CAD build for the part. Positions are in the model's coordinates, mm. Face numbers are marked on the shaded views. A direction names the side the tool comes from. Coordinates: 2 decimals unless noted, no trailing zeros. Loops run counter-clockwise (first coordinate to the right, second up) from the corner with the lowest first, then second, coordinate; pieces in that order, holes last. Notation, with made-up numbers: (-19, 74.25) -> (38, 74.25) arc R23 ccw to (38, 82.25) -> close; hole circle Ø7 at (8, -12). An arc over 180 degrees is marked (long way). Return JSON: item names as keys, results as strings. Group by question number.
(1) Probe L1, parallel to Z at x = 0, y = -0.7; L2, parallel to Z at x = 0, y = 0.6; L3, parallel to Y at x = -5, z = 0.75. List the from-to ranges inside material, lowest first.
(2) Tool access for the marked faces 4 and 5: list every direction of +Z, -Z, +X, -X, +Y, -Y with a clear straight run to the whole face (end or side of a thin tool).
(3) Mould opens along X. For the marked faces 1, 2 and 3 say: pulls with the +X half, pulls with the -X half, needs draft (parallel to the pull), parting line crosses it, or undercut.
(4) Saw through at C-C on y = 0.55. Write the cut outline in (x, z).
(5) Saw through at A-A on z = 0. Write the cut outline in (x, y).
(6) Flat gauge pins, fed straight in: pin 1 Ø1.5 at (x, y) = (-0.5, 0) entering from -Z; pin 2 Ø2 at (x, z) = (0, 0) entering from -Y. Where does each tip first touch, or does it go through?
(7) Saw through at B-B on x = 0. Write the cut outline in (y, z), then the cut area to 3 significant figures.
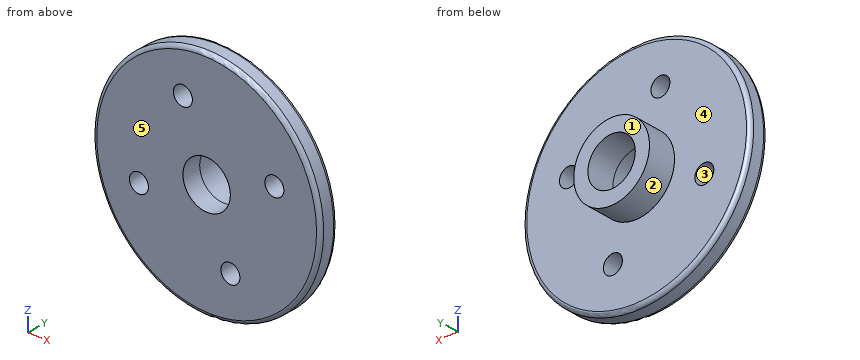
```python
from build123d import *

# Parameters (mm, degrees)
F0_R     = 6
F0_R_2   = 0.5
F0_R_3   = 1.25
F1_DEPTH = 1
F2_R     = 0.2
F3_R     = 2
F3_R_2   = 1.25
F4_DEPTH = 1.5


with BuildPart() as f1:
    # F0 (on Front) → F1 (new body)
    with BuildSketch(Plane.XZ):
        Circle(F0_R)
        with Locations((-3.573598, -1.254015)):
            Circle(F0_R_2, mode=Mode.SUBTRACT)
        with Locations((1.254015, -3.573598)):
            Circle(F0_R_2, mode=Mode.SUBTRACT)
        with Locations((-1.254015, 3.573598)):
            Circle(F0_R_2, mode=Mode.SUBTRACT)
        Circle(F0_R_3, mode=Mode.SUBTRACT)
        with Locations((3.573598, 1.254015)):
            Circle(F0_R_2, mode=Mode.SUBTRACT)
    extrude(amount=F1_DEPTH)

    # F2
    f2_edges = [f1.edges().sort_by_distance(p)[0] for p in [
        (-6, 0, 0),
        (-6, -1, 0),
    ]]
    fillet(f2_edges, radius=F2_R)

    # F3 (on face) → F4 (join)
    with BuildSketch(Plane(origin=(0, 0, 0), x_dir=(-1, 0, 0), z_dir=(0, 1, 0))):
        Circle(F3_R)
        Circle(F3_R_2, mode=Mode.SUBTRACT)
    extrude(amount=F4_DEPTH)


solid = f1.part
```
Geometry results:
{
 "1": {"L1": "-6 to -1.25, 1.25 to 6", "L2": "-2 to -1.25, 1.25 to 2", "L3": "-1 to 0"},
 "2": {"face 4": "+Y", "face 5": "+Z, -Z, +X, -X, -Y"},
 "3": {"face 1": "needs draft", "face 2": "parting line crosses it", "face 3": "undercut"},
 "4": {"outline": "circle Ø4 at (0, 0); hole circle Ø2.5 at (0, 0)"},
 "5": {"outline": "(-6, -0.8) arc R0.2 ccw to (-5.8, -1) -> (-1.25, -1) -> (-1.25, 1.5) -> (-2, 1.5) -> (-2, 0) -> (-5.8, 0) arc R0.2 ccw to (-6, -0.2) -> close; (1.25, -1) -> (5.8, -1) arc R0.2 ccw to (6, -0.8) -> (6, -0.2) arc R0.2 ccw to (5.8, 0) -> (2, 0) -> (2, 1.5) -> (1.25, 1.5) -> close"},
 "6": {"pin 1": "z = -6", "pin 2": "through"},
 "7": {"outline": "(-1, -5.8) arc R0.2 ccw to (-0.8, -6) -> (-0.2, -6) arc R0.2 ccw to (0, -5.8) -> (0, -2) -> (1.5, -2) -> (1.5, -1.25) -> (-1, -1.25) -> close; (-1, 1.25) -> (1.5, 1.25) -> (1.5, 2) -> (0, 2) -> (0, 5.8) arc R0.2 ccw to (-0.2, 6) -> (-0.8, 6) arc R0.2 ccw to (-1, 5.8) -> close", "area": "11.7 mm²"}
}
